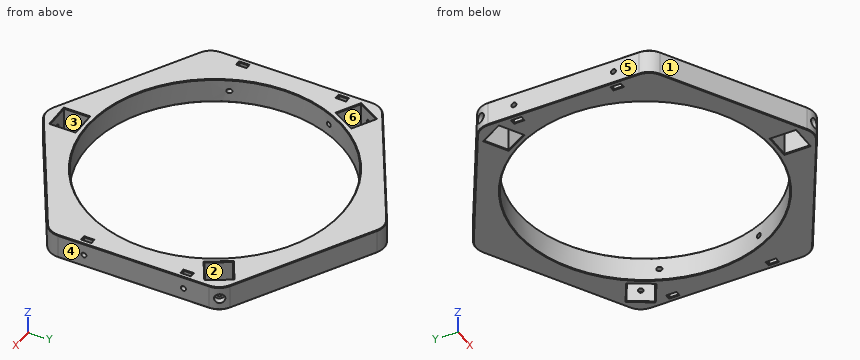
from build123d import *

# Parameters (mm, degrees)
SKETCH1_R           = 77
BOSS_EXTRUDE1_DEPTH = 15
SKETCH2_W           = 15.2
SKETCH2_H           = 15.2
CUT_EXTRUDE1_DEPTH  = 16
FILLET1_R           = 11.11
SKETCH9_R           = 1.5
CUT_EXTRUDE6_DEPTH  = 3
SKETCH10_R          = 3
CUT_EXTRUDE7_DEPTH  = 31.844449077
CIRPATTERN2_COUNT   = 3
SKETCH13_R          = 1.5
CUT_EXTRUDE10_DEPTH = 181.0000001
SKETCH14_W          = 2.5
SKETCH14_H          = 5.6
CUT_EXTRUDE11_DEPTH = 16.0000001
CHAMFER1_SIZE       = 0.4


with BuildPart() as part:
    # Sketch1 → Boss-Extrude1 (new body)
    with BuildSketch(Plane.XY):
        Polygon((0, 103.923048454), (90, 51.961524227), (90, -51.961524227), (0, -103.923048454), (-90, -51.961524227), (-90, 51.961524227), align=None)
        Circle(SKETCH1_R, mode=Mode.SUBTRACT)
    extrude(amount=BOSS_EXTRUDE1_DEPTH)

    # Sketch2 → Cut-Extrude1 (cut, through all)
    with BuildSketch(Plane.XY.offset(15)):
        with Locations((0, -87.6)):
            Rectangle(SKETCH2_W, SKETCH2_H)
        Polygon((-65.482032303, 46.581793069), (-73.082032303, 33.418206931), (-86.24561844, 41.018206931), (-78.64561844, 54.181793069), align=None)
        Polygon((73.082032303, 33.418206931), (65.482032303, 46.581793069), (78.64561844, 54.181793069), (86.24561844, 41.018206931), align=None)
    extrude(amount=-CUT_EXTRUDE1_DEPTH, mode=Mode.SUBTRACT)

    # Fillet1
    fillet1_edges = [part.edges().sort_by_distance(p)[0] for p in [
        (0, -103.923048454, 7.5),
        (-90, -51.961524227, 7.5),
        (-90, 51.961524227, 7.5),
        (0, 103.923048454, 7.5),
        (90, 51.961524227, 7.5),
        (90, -51.961524227, 7.5),
    ]]
    fillet(fillet1_edges, radius=FILLET1_R)

    # Sketch9 → Cut-Extrude6 (cut)
    with BuildSketch(Plane(origin=(-82.44561844, 47.6, 0), x_dir=(0, 0, -1), z_dir=(0.866025404, -0.5, 0))):
        with Locations((-7.5, 0)):
            Circle(SKETCH9_R)
    cut_extrude6 = extrude(amount=-CUT_EXTRUDE6_DEPTH, mode=Mode.SUBTRACT)

    # Sketch10 → Cut-Extrude7 (cut, through all)
    with BuildSketch(Plane(origin=(-85.043694652, 49.1, 0), x_dir=(0, 0, -1), z_dir=(0.866025404, -0.5, 0))):
        with Locations((-7.5, 0)):
            Circle(SKETCH10_R)
    cut_extrude7 = extrude(amount=-CUT_EXTRUDE7_DEPTH, mode=Mode.SUBTRACT)

    # CirPattern2: Cut-Extrude6, Cut-Extrude7 ×3 about axis
    cirpattern2_axis = Axis((0, 0, 0), (0, 0, 1))
    for i in range(1, CIRPATTERN2_COUNT):
        add(cut_extrude6.rotate(cirpattern2_axis, i * 360 / CIRPATTERN2_COUNT), mode=Mode.SUBTRACT)
        add(cut_extrude7.rotate(cirpattern2_axis, i * 360 / CIRPATTERN2_COUNT), mode=Mode.SUBTRACT)

    # Sketch13 → Cut-Extrude10 (cut, through all)
    with BuildSketch(Plane.ZY.offset(90)):
        with Locations((7.5, -30)):
            Circle(SKETCH13_R)
        with Locations((7.5, 30)):
            Circle(SKETCH13_R)
    extrude(amount=-CUT_EXTRUDE10_DEPTH, mode=Mode.SUBTRACT)

    # Sketch14 → Cut-Extrude11 (cut, through all)
    with BuildSketch(Plane.XY.offset(15)):
        with Locations((-85.75, 30)):
            Rectangle(SKETCH14_W, SKETCH14_H)
        with Locations((-85.75, -30)):
            Rectangle(SKETCH14_W, SKETCH14_H)
        with Locations((85.75, -30)):
            Rectangle(SKETCH14_W, SKETCH14_H)
        with Locations((85.75, 30)):
            Rectangle(SKETCH14_W, SKETCH14_H)
    extrude(amount=-CUT_EXTRUDE11_DEPTH, mode=Mode.SUBTRACT)

    # Chamfer1
    chamfer1_edges = [part.edges().sort_by_distance(p)[0] for p in [
        (-77, 0, 0),
        (-77, 0, 15),
        (87, 30, 0),
        (84.5, 30, 0),
        (85.75, 32.8, 0),
        (85.75, 27.2, 0),
        (85.75, 32.8, 15),
        (84.5, 30, 15),
        (85.75, 27.2, 15),
        (87, 30, 15),
        (87, -30, 0),
        (84.5, -30, 0),
        (85.75, -32.8, 0),
        (85.75, -27.2, 0),
        (87, -30, 15),
        (85.75, -27.2, 15),
        (84.5, -30, 15),
        (85.75, -32.8, 15),
        (-87, -30, 0),
        (-84.5, -30, 0),
        (-85.75, -32.8, 0),
        (-85.75, -27.2, 0),
        (-85.75, -32.8, 15),
        (-84.5, -30, 15),
        (-85.75, -27.2, 15),
        (-87, -30, 15),
        (-87, 30, 0),
        (-84.5, 30, 0),
        (-85.75, 32.8, 0),
        (-85.75, 27.2, 0),
        (-87, 30, 15),
        (-85.75, 27.2, 15),
        (-84.5, 30, 15),
        (-85.75, 32.8, 15),
        (7.6, -87.6, 0),
        (0, -95.2, 0),
        (-7.6, -87.6, 0),
        (0, -80, 0),
        (7.6, -87.6, 15),
        (0, -80, 15),
        (-7.6, -87.6, 15),
        (0, -95.2, 15),
        (-79.663825372, 37.218206931, 0),
        (-82.44561844, 47.6, 0),
        (-72.063825372, 50.381793069, 0),
        (-69.282032303, 40, 0),
        (-79.663825372, 37.218206931, 15),
        (-69.282032303, 40, 15),
        (-72.063825372, 50.381793069, 15),
        (-82.44561844, 47.6, 15),
        (72.063825372, 50.381793069, 0),
        (82.44561844, 47.6, 0),
        (79.663825372, 37.218206931, 0),
        (69.282032303, 40, 0),
        (72.063825372, 50.381793069, 15),
        (69.282032303, 40, 15),
        (79.663825372, 37.218206931, 15),
        (82.44561844, 47.6, 15),
        (-45, -77.942286341, 0),
        (-45, -77.942286341, 15),
        (45, -77.942286341, 0),
        (-90, 0, 0),
        (-45, 77.942286341, 0),
        (45, 77.942286341, 0),
        (90, 0, 0),
        (0, -102.204325473, 0),
        (88.511542236, -51.102162736, 0),
        (88.511542236, 51.102162736, 0),
        (0, 102.204325473, 0),
        (-88.511542236, 51.102162736, 0),
        (-88.511542236, -51.102162736, 0),
        (-90, 0, 15),
        (45, -77.942286341, 15),
        (90, 0, 15),
        (45, 77.942286341, 15),
        (-45, 77.942286341, 15),
        (0, -102.204325473, 15),
        (88.511542236, -51.102162736, 15),
        (88.511542236, 51.102162736, 15),
        (0, 102.204325473, 15),
        (-88.511542236, 51.102162736, 15),
        (-88.511542236, -51.102162736, 15),
    ]]
    chamfer(chamfer1_edges, length=CHAMFER1_SIZE)


solid = part.part
Could you check a few things on this model? Use its own coordinates, in mm. Face numbers are marked on the shaded views. A direction names the side the tool comes from. Round coordinates to 2 decimals unless told otherwise and drop trailing zeros. Order: outer loops, then holes, each group sorted by start corner. A loop starts at its lowest first (then second) coordinate and runs counter-clockwise, first axis right, second up. Notation, with made-up numbers: M 15.5,44 L 31.5,44 A27 cw 31.5,77 Z; hole C -34,-17 d1. An arc over 180 degrees is marked long. One line per item, written item: value.
(1) Imagine slicing it at B-B (y = -82.5). Write out the boundary of the cut face in (x, z), and give its area (3 significant figures).
Ans:
outline: M -37.11,0.4 L -36.31,0 L -8,0 L -7.6,0.4 L -7.6,14.6 L -8,15 L -36.31,15 L -37.11,14.6 Z; M 7.6,0.4 L 8,0 L 36.31,0 L 37.11,0.4 L 37.11,14.6 L 36.31,15 L 8,15 L 7.6,14.6 Z
area: 884 mm^2
(2) I'm going to push flat-ended pins straight in: P1, Ø6, axis at y = -30, z = 6.5, coming from the -X side; P2, Ø1.5, axis at x = -26, z = 10, coming from the +Y side; P3, Ø1, axis at x = -39.5, z = 12, coming from the -Y side; P4, Ø1.2, axis at x = 85.5, z = 8, coming from the +Y side. Where does each tip first touch, or does it pass through?
Ans:
P1: stops at x = -90
P2: stops at y = 89.34
P3: stops at y = -81.41
P4: stops at y = 54.89
(3) Imagine slicing it at A-A (y = 0). Write out the boundary of the cut face in (x, z).
Ans:
outline: M -90,0.4 L -89.6,0 L -77.4,0 L -77,0.4 L -77,14.6 L -77.4,15 L -89.6,15 L -90,14.6 Z; M 77,0.4 L 77.4,0 L 89.6,0 L 90,0.4 L 90,14.6 L 89.6,15 L 77.4,15 L 77,14.6 Z
(4) If we mould it in two halves opening along X, with no side actions, what happens to the marked faces 1, 2, 3 and 4? For each: released by +X, released by -X, zero draft, split by the parting line, or undercut.
Ans:
face 1: released by -X
face 2: undercut
face 3: undercut
face 4: released by +X
(5) Which directions (+Z, -Z, +X, -X, +Y, -Y) give clear straight access to the entire face, cutting with the end or side of a thin tool? Please do the marked faces 5 and 6.
Ans:
face 5: +Z, -Z, -X, +Y, -Y
face 6: +Z, -Z
(6) I need wall thicknesses on line 1 along Z through (x, y) = (79, -30); line 2 along Y through (x, z) = (78.5, 7.5); line 3 along Y through (x, z) = (-87.95, 7.5). Which ranges of each line are inside material? Lowest first, please. Write a range as from..to.
Ans:
line 1: z = 0..6, 9..15
line 2: y = -58.6..-31.5, -28.5..28.5, 31.5..36.55, 54.1..58.6
line 3: y = -51.98..-31.5, -28.5..28.5, 31.5..47.31
